Check sheet for the modelled part. Datum: model origin and axes. Units: mm. Face numbers are marked on the shaded views. A direction names the side the tool comes from. Round coordinates to 2 decimals unless told otherwise and drop trailing zeros. Write each loop counter-clockwise with the first axis right and the second up, starting at its lowest first coordinate (ties: lowest second). Pieces come first, ordered by that corner, then holes. Notation, with made-up numbers: (-36.5, -23.75) -> (-8.5, -23.75) arc R18 cw to (-8.5, 7.25) -> close; hole circle Ø8 at (-32.5, 28). An arc over 180 degrees is marked (long way). One line per item, written item: value.
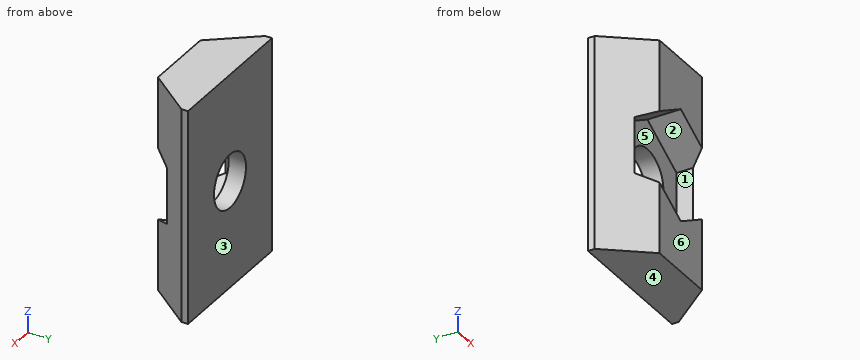
from build123d import *

# Parameters (mm, degrees)
RESSALTO_EXTRUS_O1_DEPTH   = 16
CORTE_EXTRUS_O1_DEPTH      = 18.262748912
CORTE_EXTRUS_O1_DEPTH_BACK = 18.262748912
ESBO_O2_R                  = 2
CORTE_EXTRUS_O2_DEPTH      = 2.5


with BuildPart() as part:
    # Esboço1 → Ressalto-extrusão1 (new body)
    with BuildSketch(Plane.XY):
        Polygon((-2.65, 0), (2.65, 0), (5.25, 3.3), (5.25, 3.8), (-5.25, 3.8), (-5.25, 3.3), align=None)
    extrude(amount=RESSALTO_EXTRUS_O1_DEPTH)

    # Esboço2 → Corte-extrusão1 (cut, two sides: drawn at the far end of the back side and taken through both)
    with BuildSketch(Plane(origin=(0, 3.8, 0), x_dir=(1, 0, 0), z_dir=(0, 1, 0)).offset(-CORTE_EXTRUS_O1_DEPTH_BACK)):
        with Locations(Location((0, -8, 0), (0, 0, 270))):
            Circle(ESBO_O2_R)
    extrude(amount=CORTE_EXTRUS_O1_DEPTH + CORTE_EXTRUS_O1_DEPTH_BACK, mode=Mode.SUBTRACT)

    # Esboço3 → Corte-extrusão2 (cut)
    with BuildSketch(Plane.XZ):
        Polygon((0, 12.214656965), (-3.65, 10.107328483), (-3.65, 5.892671517), (0, 3.785343035), (3.65, 5.892671517), (3.65, 10.107328483), align=None)
    extrude(amount=-CORTE_EXTRUS_O2_DEPTH, mode=Mode.SUBTRACT)


solid = part.part
Item 1: Sectioned sample at D-D (y = 2). Enter the section's corners in (x, z).
Result set:
outline: (-4.23, 0) -> (4.23, 0) -> (4.23, 16) -> (-4.23, 16) -> close; hole (-3.65, 5.89) -> (0, 3.79) -> (3.65, 5.89) -> (3.65, 10.11) -> (0, 12.21) -> (-3.65, 10.11) -> close
Item 2: Sectioned sample at A-A (z = 8). Enter the section's corners in (x, y).
Result set:
outline: (-5.25, 3.3) -> (-3.65, 1.27) -> (-3.65, 2.5) -> (-2, 2.5) -> (-2, 3.8) -> (-5.25, 3.8) -> close; (2, 2.5) -> (3.65, 2.5) -> (3.65, 1.27) -> (5.25, 3.3) -> (5.25, 3.8) -> (2, 3.8) -> close
Item 3: Material ranges on line 1 along Z through (x, y) = (0, 3.3); line 2 along X through (y, z) = (3.55, 8); line 3 along X through (y, z) = (3.15, 8), recorded low to high.
Result set:
line 1: 0 to 6, 10 to 16
line 2: -5.25 to -2, 2 to 5.25
line 3: -5.13 to -2, 2 to 5.13
Item 4: Depth check by flat-ended pin: pin 1 (2 mm diameter, centred on x = -0.5, y = 2.5, fed in from -Z); pin 2 (1 mm diameter, centred on y = 2, z = 7, fed in from -X); pin 3 (3 mm diameter, centred on x = 0, z = 8, fed in from -Y); pin 4 (1.4 mm diameter, centred on y = 2, z = 7.5, fed in from +X). Enter the tip coordinate at first touch or a pass-through.
Result set:
pin 1: z = 0
pin 2: x = -4.62
pin 3: through
pin 4: x = 4.78
Item 5: Sectioned sample at C-C (x = -1.5). Enter the section's corners in (y, z), then the cut area to 3 significant figures.
Result set:
outline: (0, 0) -> (3.8, 0) -> (3.8, 6.68) -> (2.5, 6.68) -> (2.5, 4.65) -> (0, 4.65) -> close; (0, 11.35) -> (2.5, 11.35) -> (2.5, 9.32) -> (3.8, 9.32) -> (3.8, 16) -> (0, 16) -> close
area: 40.6 mm^2
Item 6: Sectioned sample at B-B (y = 0.8). Enter the section's corners in (x, z).
Result set:
outline: (-3.28, 0) -> (3.28, 0) -> (3.28, 5.68) -> (0, 3.79) -> (-3.28, 5.68) -> close; (-3.28, 10.32) -> (0, 12.21) -> (3.28, 10.32) -> (3.28, 16) -> (-3.28, 16) -> close
Item 7: Tool access check on the marked faces 5 and 6. Record the directions out of +Z, -Z, +X, -X, +Y, -Y that give a thin tool (end or side, any length) a straight path to the whole face; none if there is none.
Result set:
face 5: -Y
face 6: +Z, -Z, +X, -X, -Y
Item 8: Release check for a two-part mould opening along Z. For the marked faces 1, 2, 3 and 4 record: pulls with the +Z half, pulls with the -Z half, needs draft (parallel to the pull), parting line crosses it, or undercut.
Result set:
face 1: undercut
face 2: undercut
face 3: needs draft
face 4: pulls with the -Z half
